For this review, take the finished solid that the model builds, in its own axes (mm). Face numbers are marked on the shaded views. A direction names the side the tool comes from. Give positions to 0.01 mm unless a question says otherwise; leave off trailing zeros. Loops run counter-clockwise (first coordinate to the right, second up) from the corner with the lowest first, then second, coordinate; pieces in that order, holes last.
```python
from build123d import *

# Parameters (mm, degrees)
SKETCH1_W           = 78
SKETCH1_H           = 41
SKETCH1_R           = 5
BOSS_EXTRUDE1_DEPTH = 7
BOSS_EXTRUDE3_START = -41
BOSS_EXTRUDE3_DEPTH = 7
BOSS_EXTRUDE6_DEPTH = 7
SKETCH10_W          = 66.063477679
SKETCH10_H          = 45
BOSS_EXTRUDE7_DEPTH = 7


with BuildPart() as part:
    # Sketch1 → Boss-Extrude1 (new body)
    with BuildSketch(Plane(origin=(0, 0, 0), x_dir=(1, 0, 0), z_dir=(0, 1, 0))):
        with Locations((39, 20.5)):
            Rectangle(SKETCH1_W, SKETCH1_H)
        with Locations(Location((20, 12, 0), (0, 0, 270))):
            Circle(SKETCH1_R, mode=Mode.SUBTRACT)
        with Locations(Location((58, 12, 0), (0, 0, 270))):
            Circle(SKETCH1_R, mode=Mode.SUBTRACT)
    extrude(amount=BOSS_EXTRUDE1_DEPTH)

    # Sketch5 → Boss-Extrude3 (add)
    with BuildSketch(Plane.XY.offset(BOSS_EXTRUDE3_START)):
        Polygon((0, 7), (0, 76.371997336), (78, 40), (78, 7), align=None)
    extrude(amount=BOSS_EXTRUDE3_DEPTH)

    # Sketch6 → Boss-Extrude6 (add)
    with BuildSketch(Plane(origin=(0, 0, 0), x_dir=(0, 0, -1), z_dir=(1, 0, 0))):
        Polygon((34, 7), (34, 32), (0, 7), align=None)
    extrude(amount=BOSS_EXTRUDE6_DEPTH)

    # Sketch10 → Boss-Extrude7 (add)
    with BuildSketch(Plane(origin=(29.252172085, 62.731485475, 0), x_dir=(0.9063077870366529, -0.4226182617406933, 0), z_dir=(0.4226182617406933, 0.9063077870366529, 0))):
        with Locations((10.755538079, 63.5)):
            Rectangle(SKETCH10_W, SKETCH10_H)
        with BuildLine():
            Line((-6.212723081, 70), (15.725019171, 70))
            ThreePointArc((15.725019171, 70), (32.787276919, 66), (15.725019171, 62))
            Line((15.725019171, 62), (-6.212723081, 62))
            ThreePointArc((-6.212723081, 62), (-10.212723081, 66), (-6.212723081, 70))
        make_face(mode=Mode.SUBTRACT)
    extrude(amount=-BOSS_EXTRUDE7_DEPTH)


solid = part.part
```
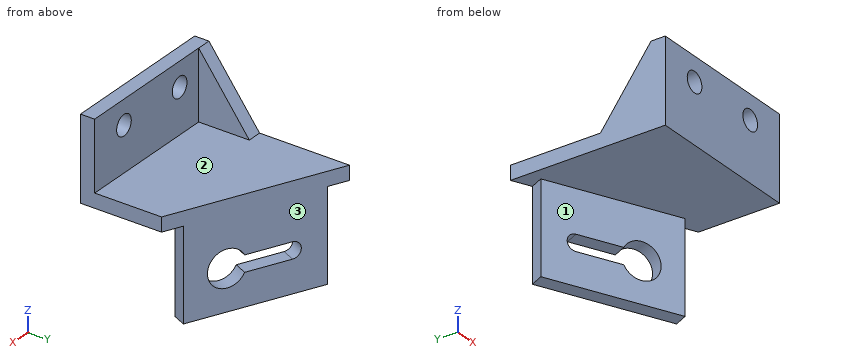
Q1. Machinability: for the marked faces 1, 2 and 3, which of the approach directions +Z, -Z, +X, -X, +Y, -Y give a long, thin tool a straight path to every point of the face, cutting with its end or side? Answer none if there is none.
Answers:
face 1: -Z, -X, -Y
face 2: +Z, +X, +Y
face 3: +Z, -Z, +X, +Y
Q2. Consider section C-C on z = -67.5. Give the boundary of the cut face in (x, y), plus the area to 3 significant figures.
Answers:
outline: (6.1, 65.8) - (17.3, 60.58) - (20.26, 66.92) - (9.06, 72.15) - close; (55.9, 42.58) - (65.98, 37.88) - (68.94, 44.23) - (58.85, 48.93) - close
area: 164 mm2
Q3. For probe 1 along X at (y, z) = (3.5, -12); probe 2 along Y at (x, z) = (64, -23.5); probe 3 along Z at (x, y) = (8, 40.5), list the stretches that pass through material, from the lowest coordinate up.
Answers:
probe 1: x = 0 to 15, 25 to 53, 63 to 78
probe 2: y = 0 to 7
probe 3: z = -41 to -34
Q4. Consider section B-B on z = -12. Give the boundary of the cut face in (x, y), plus the area to 3 significant figures.
Answers:
outline: (0, 0) - (15, 0) - (15, 7) - (7, 7) - (7, 15.82) - (0, 15.82) - close; (25, 0) - (53, 0) - (53, 7) - (25, 7) - close; (63, 0) - (78, 0) - (78, 7) - (63, 7) - close
area: 468 mm2
Q5. For pin 1 Ø1.5 at (x, z) = (50, -33) entering from +Y; pin 2 Ø2 at (x, z) = (64.5, -37) entering from +Y; pin 3 Ø10 at (x, y) = (18, 34.5) entering from -Z, all flat-tipped, find the tip position at first contact; note any pin that passes through.
Answers:
pin 1: stops at y = 7
pin 2: stops at y = 46.76
pin 3: stops at z = -41
Q6. Consider section A-A on x = 30. Give the boundary of the cut face in (y, z).
Answers:
outline: (0, -41) - (54.66, -41) - (54.66, -62) - (62.38, -62) - (62.38, -34) - (7, -34) - (7, 0) - (0, 0) - close; (54.66, -86) - (62.38, -86) - (62.38, -70) - (54.66, -70) - close
Q7. Consider section D-D on x = 11. Give the boundary of the cut face in (y, z), plus the area to 3 significant figures.
Answers:
outline: (0, -41) - (63.52, -41) - (63.52, -86) - (71.24, -86) - (71.24, -34) - (7, -34) - (7, 0) - (0, 0) - close
area: 1,080 mm2
